Geometry check sheet. Reference: the model listing, model coordinates, mm. Coordinates: 2 decimals unless noted, no trailing zeros. Order: outer loops, then holes, each group sorted by start corner. A loop starts at its lowest first (then second) coordinate and runs counter-clockwise, first axis right, second up. Notation, with made-up numbers: (-30.5, 36) - (14.5, 36) arc R9 ccw to (14.5, 51) - close; hole circle Ø10 at (15, 11.25). An arc over 180 degrees is marked (long way). Return JSON: item names as keys, results as strings. Group by question number.
Item 1: Section check C-C on y = 95. Enter the section's corners in (x, z).
Item 2: Section check D-D on x = 29.5. Enter the section's corners in (y, z), then the cut area to 3 significant figures.
Item 3: Scan lines: probe 1 along Y at (x, z) = (3, 4.25); probe 2 along X at (y, z) = (105, 6); probe 3 along X at (y, z) = (20, 6). Record each from-to range of solid material in increasing order.
Item 4: Gauge pin test, flat ends, axial feed: pin 1 (2 mm diameter, centred on x = 33, z = 1, fed in from -Y); pin 2 (1 mm diameter, centred on y = 2, z = 5.5, fed in from +X); pin 3 (2.5 mm diameter, centred on x = 177.5, y = 3, fed in from -Z); pin 4 (1.5 mm diameter, centred on x = 94.5, y = 11, fed in from +Z). Record the tip position at first contact, or that the pin passes through.
Item 5: Section check A-A on x = 110. Enter the section's corners in (y, z), then the cut area to 3 significant figures.
Item 6: Section check B-B on z = 5.75. Enter the section's corners in (x, y), then the cut area to 3 significant figures.
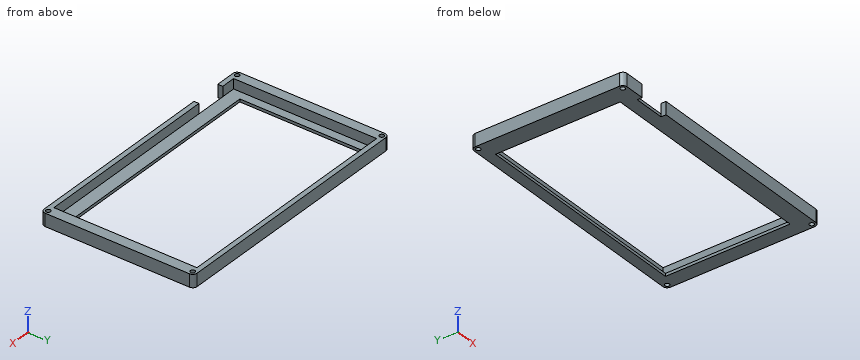
from build123d import *

# Parameters (mm, degrees)
SKETCH_1_R          = 1.6
EXTRUDE_3_DEPTH     = 9
SKETCH_3_W          = 166
SKETCH_3_H          = 101
CUT_EXTRUDE_1_DEPTH = 7
SKETCH_5_W          = 157
SKETCH_5_H          = 88
CUT_EXTRUDE_2_DEPTH = 211.459616079
SKETCH_6_W          = 22
SKETCH_6_H          = 3.5
CUT_EXTRUDE_3_DEPTH = 211.535626439


with BuildPart() as part:
    # 草图1 → 凸台-拉伸3 (new body)
    with BuildSketch(Plane.XY):
        with BuildLine():
            Line((3, 0), (177.5, 0))
            ThreePointArc((177.5, 0), (179.621320344, 0.878679656), (180.5, 3))
            Line((180.5, 3), (180.5, 105))
            ThreePointArc((180.5, 105), (179.621320344, 107.121320344), (177.5, 108))
            Line((177.5, 108), (3, 108))
            ThreePointArc((3, 108), (0.878679656, 107.121320344), (0, 105))
            Line((0, 105), (0, 3))
            ThreePointArc((0, 3), (0.878679656, 0.878679656), (3, 0))
        make_face()
        with Locations((3, 3)):
            Circle(SKETCH_1_R, mode=Mode.SUBTRACT)
        with Locations((3, 105)):
            Circle(SKETCH_1_R, mode=Mode.SUBTRACT)
        with Locations((177.5, 105)):
            Circle(SKETCH_1_R, mode=Mode.SUBTRACT)
        with Locations((177.5, 3)):
            Circle(SKETCH_1_R, mode=Mode.SUBTRACT)
    extrude(amount=EXTRUDE_3_DEPTH)

    # 草图3 → 切除-拉伸1 (cut)
    with BuildSketch(Plane.XY.offset(9)):
        with Locations((90, 54)):
            Rectangle(SKETCH_3_W, SKETCH_3_H)
    extrude(amount=-CUT_EXTRUDE_1_DEPTH, mode=Mode.SUBTRACT)

    # 草图5 → 切除-拉伸2 (cut, through all)
    with BuildSketch(Plane.XY.offset(2)):
        with Locations((91.5, 56.5)):
            Rectangle(SKETCH_5_W, SKETCH_5_H)
    extrude(amount=-CUT_EXTRUDE_2_DEPTH, mode=Mode.SUBTRACT)

    # 草图6 → 切除-拉伸3 (cut, through all)
    with BuildSketch(Plane.XY.offset(9)):
        with Locations((28, 1.75)):
            Rectangle(SKETCH_6_W, SKETCH_6_H)
    extrude(amount=-CUT_EXTRUDE_3_DEPTH, mode=Mode.SUBTRACT)


solid = part.part
Computed:
{
 "1": {"outline": "(0, 0) - (13, 0) - (13, 2) - (7, 2) - (7, 9) - (0, 9) - close; (170, 0) - (180.5, 0) - (180.5, 9) - (173, 9) - (173, 2) - (170, 2) - close"},
 "2": {"outline": "(3.5, 0) - (12.5, 0) - (12.5, 2) - (3.5, 2) - close; (100.5, 0) - (108, 0) - (108, 9) - (104.5, 9) - (104.5, 2) - (100.5, 2) - close", "area": "57.5 mm²"},
 "3": {"probe 1": "y = 0 to 1.4, 4.6 to 103.4, 106.6 to 108", "probe 2": "x = 0 to 1.4, 4.6 to 175.9, 179.1 to 180.5", "probe 3": "x = 0 to 7, 173 to 180.5"},
 "4": {"pin 1": "stops at y = 3.5", "pin 2": "stops at x = 180.46", "pin 3": "passes through", "pin 4": "stops at z = 2"},
 "5": {"outline": "(0, 0) - (12.5, 0) - (12.5, 2) - (3.5, 2) - (3.5, 9) - (0, 9) - close; (100.5, 0) - (108, 0) - (108, 9) - (104.5, 9) - (104.5, 2) - (100.5, 2) - close", "area": "89.0 mm²"},
 "6": {"outline": "(0, 3) arc R3 ccw to (3, 0) - (17, 0) - (17, 3.5) - (7, 3.5) - (7, 104.5) - (173, 104.5) - (173, 3.5) - (39, 3.5) - (39, 0) - (177.5, 0) arc R3 ccw to (180.5, 3) - (180.5, 105) arc R3 ccw to (177.5, 108) - (3, 108) arc R3 ccw to (0, 105) - close; hole circle Ø3.2 at (3, 3); hole circle Ø3.2 at (3, 105); hole circle Ø3.2 at (177.5, 3); hole circle Ø3.2 at (177.5, 105)", "area": "2,610 mm²"}
}
